```python
from build123d import *
from OCP.BRepFilletAPI import BRepFilletAPI_MakeChamfer

# Parameters (mm, degrees)
SKETCH2_R                = 12
BOSS_EXTRUDE1_DEPTH      = 81.85
SKETCH3_W                = 28.5
SKETCH3_H                = 57
SKETCH3_R                = 1.5
BOSS_EXTRUDE2_DEPTH      = 3
CHAMFER1_SIZE            = 1.5
SKETCH4_R                = 9.4
BOSS_EXTRUDE3_DEPTH      = 25.1
CUT_EXTRUDE1_DEPTH       = 88.8335642
CUT_EXTRUDE1_DEPTH_BACK  = 88.8335642
CHAMFER2_SIZE            = 2
CHAMFER2_SIZE2           = 2.066892656
CHAMFER3_SIZE            = 2
SKETCH6_R                = 4.5
CUT_EXTRUDE2_DEPTH       = 88.8335642
CUT_EXTRUDE2_DEPTH_BACK  = 88.8335642
SKETCH7_W                = 35.652875986
SKETCH7_H                = 43.298184849
SKETCH7_W_2              = 11
SKETCH7_H_2              = 30
CUT_EXTRUDE3_DEPTH       = 44
SKETCH8_R                = 4.5
BOSS_EXTRUDE4_DEPTH      = 2.5
BOSS_EXTRUDE4_DEPTH_BACK = 2.5
SKETCH9_R                = 3.5
CUT_EXTRUDE4_DEPTH       = 89.891703775


with BuildPart() as part:
    # Sketch2 → Boss-Extrude1 (new body)
    with BuildSketch(Plane.XY):
        Circle(SKETCH2_R)
    extrude(amount=-BOSS_EXTRUDE1_DEPTH)

    # Sketch3 → Boss-Extrude2 (add)
    with BuildSketch(Plane.XY):
        Rectangle(SKETCH3_W, SKETCH3_H)
        with Locations((0, 20.5)):
            Circle(SKETCH3_R, mode=Mode.SUBTRACT)
        with Locations((0, -20.5)):
            Circle(SKETCH3_R, mode=Mode.SUBTRACT)
    extrude(amount=BOSS_EXTRUDE2_DEPTH)

    # Chamfer1
    chamfer1_edges = [part.edges().sort_by_distance(p)[0] for p in [
        (-1.5, 20.5, 3),
        (-1.5, -20.5, 3),
    ]]
    chamfer(chamfer1_edges, length=CHAMFER1_SIZE)

    # Sketch4 → Boss-Extrude3 (add)
    with BuildSketch(Plane.XY.offset(3)):
        Circle(SKETCH4_R)
    extrude(amount=BOSS_EXTRUDE3_DEPTH)

    # Sketch5 → Cut-Extrude1 (cut, two sides)
    with BuildSketch(Plane(origin=(0, 0, 0), x_dir=(1, 0, 0), z_dir=(0, 1, 0))) as cut_extrude1_sk:
        Polygon((-7.85, -3), (-7.05, -28.1), (-9.4, -28.1), (-9.4, -3), align=None)
        Polygon((9.4, -3), (7.85, -3), (7.05, -28.1), (9.4, -28.1), align=None)
    extrude(amount=CUT_EXTRUDE1_DEPTH, mode=Mode.SUBTRACT)
    extrude(cut_extrude1_sk.sketch, amount=-CUT_EXTRUDE1_DEPTH_BACK, mode=Mode.SUBTRACT)

    # Chamfer2: one chamfer whose edges measure the first distance from different faces: ONE call of the kernel's chamfer builder (chamfer() names one face for all edges)
    chamfer2_edges_1 = [part.edges().sort_by_distance(p)[0] for p in [
        (0, -9.4, 28.1),
        (0, 9.4, 28.1),
    ]]
    chamfer2_edges_2 = [part.edges().sort_by_distance(p)[0] for p in [
        (7.05, 0, 28.1),
        (-7.05, 0, 28.1),
    ]]
    chamfer2_side_2 = [part.faces().sort_by_distance(p)[0] for p in [
        (0, 0, 28.1),
    ]]
    chamfer2 = BRepFilletAPI_MakeChamfer(part.part.solid().wrapped)
    for e in chamfer2_edges_1:
        chamfer2.Add(CHAMFER2_SIZE, e.wrapped)
    for e in chamfer2_edges_2:
        chamfer2.Add(CHAMFER2_SIZE, CHAMFER2_SIZE2, e.wrapped, chamfer2_side_2[0].wrapped)  # the first distance lies on this face
    add(Compound.cast(chamfer2.Shape()), mode=Mode.REPLACE)

    # Chamfer3
    chamfer3_edges = [part.edges().sort_by_distance(p)[0] for p in [
        (-12, 0, -81.85),
    ]]
    chamfer(chamfer3_edges, length=CHAMFER3_SIZE)

    # Sketch6 → Cut-Extrude2 (cut, two sides)
    with BuildSketch(Plane(origin=(0, 0, 0), x_dir=(0, 0, -1), z_dir=(1, 0, 0))) as cut_extrude2_sk:
        with Locations((57, -7)):
            Circle(SKETCH6_R)
    extrude(amount=CUT_EXTRUDE2_DEPTH, mode=Mode.SUBTRACT)
    extrude(cut_extrude2_sk.sketch, amount=-CUT_EXTRUDE2_DEPTH_BACK, mode=Mode.SUBTRACT)

    # Sketch7 → Cut-Extrude3 (cut)
    with BuildSketch(Plane(origin=(0, 0, -81.85), x_dir=(-1, 0, 0), z_dir=(0, 0, -1))):
        with Locations((0.794809337, 0.340632573)):
            Rectangle(SKETCH7_W, SKETCH7_H)
        Rectangle(SKETCH7_W_2, SKETCH7_H_2, mode=Mode.SUBTRACT)
    extrude(amount=-CUT_EXTRUDE3_DEPTH, mode=Mode.SUBTRACT)

    # Sketch8 → Boss-Extrude4 (add, two sides)
    with BuildSketch(Plane(origin=(0, 0, 0), x_dir=(0, 0, -1), z_dir=(1, 0, 0))) as boss_extrude4_sk:
        with Locations((57, -7)):
            Circle(SKETCH8_R)
        Polygon((55.9, -5.9), (55.9, -3.6), (58.1, -3.6), (58.1, -5.9), (60.4, -5.9), (60.4, -8.1), (58.1, -8.1), (58.1, -10.4), (55.9, -10.4), (55.9, -8.1), (53.6, -8.1), (53.6, -5.9), align=None, mode=Mode.SUBTRACT)
    extrude(amount=BOSS_EXTRUDE4_DEPTH)
    extrude(boss_extrude4_sk.sketch, amount=-BOSS_EXTRUDE4_DEPTH_BACK)

    # Sketch9 → Cut-Extrude4 (cut, through all)
    with BuildSketch(Plane(origin=(5.5, 0, 0), x_dir=(0, 0, -1), z_dir=(1, 0, 0))):
        with Locations(Location((44.65, -4, 0), (0, 0, 90))):
            Circle(SKETCH9_R)
        with Locations(Location((69.35, -4, 0), (0, 0, 90))):
            Circle(SKETCH9_R)
    extrude(amount=-CUT_EXTRUDE4_DEPTH, mode=Mode.SUBTRACT)


solid = part.part
```
Check sheet for the modelled part. Datum: model origin and axes. Units: mm. A direction names the side the tool comes from. Round coordinates to 2 decimals unless told otherwise and drop trailing zeros. Loops run counter-clockwise (first coordinate to the right, second up) from the corner with the lowest first, then second, coordinate; pieces in that order, holes last. Notation, with made-up numbers: (79.25, 13) - (100.25, 13) arc R38 cw to (100.25, 51) - close; hole circle Ø8 at (1.25, 42). An arc over 180 degrees is marked (long way). Answer as a JSON object with one key per item and string values. Group by question number.
Q1. Mould release check, pull along Y, two halves, no side actions. Record for faces 1 (the face through (-3.98, -2.54, -56.41)), 2 (the face through (-14.25, 0, 1)), 3 (the face through (0.1, 9.4, 14.4)): released by +Y, released by -Y, zero draft, split by the parting line, or undercut.
Q2. Gauge pin test, flat ends, axial feed: P1, Ø4, axis at x = -6, y = -4.5, coming from the -Z side; P2, Ø17, axis at y = -1.5, z = -59.5, coming from the -X side; P3, Ø3, axis at x = -6, z = -18, coming from the +Y side; P4, Ø1.8, axis at x = 1, y = -10, coming from the +Z side. Record the tip position at first contact, or that the pin passes through.
Q3. Set-up check for faces 4 (the face through (0, -7, -53.6)), 5 (the face through (-11.99, 0.53, -21.62)), 6 (the face through (-0.1, -9.4, 14.4)): record each of +Z, -Z, +X, -X, +Y, -Y from which the full face is reachable in a straight line by a thin tool's end or side.
Q4. Sectioned sample at A-A, the plane y = 20.5. Enter the section's corners in (x, z).
Q5. Sectioned sample at D-D, the plane z = -33.5. Enter the section's corners in (x, y), plus the area to 3 significant figures.
Q6. Sectioned sample at C-C, the plane x = 0. Count the separate pieces of the cut face and the enclosed holes in it, plus the area to 3 significant figures.
Q7. Sectioned sample at B-B, the plane z = -69.35. Enter the section's corners in (x, y), plus the area to 3 significant figures.
Q8. Scan lines: line 1 along Y through (x, z) = (0, 0.65); line 2 along Z through (x, y) = (-4.15, -7); line 3 along Z through (x, y) = (3, -4). Record each from-to range of solid material in increasing order. Write a range as [from, to].
Solution:
{
 "1": {"face 1": "undercut", "face 2": "zero draft", "face 3": "released by +Y"},
 "2": {"P1": "stops at z = -81.85", "P2": "stops at x = -5.5", "P3": "stops at y = 11.12", "P4": "stops at z = 26.35"},
 "3": {"face 4": "+X, -X", "face 5": "-Z", "face 6": "+Z, -Y"},
 "4": {"outline": "(-14.25, 0) - (-1.5, 0) - (-1.5, 1.5) - (-3, 3) - (-14.25, 3) - close; (1.5, 0) - (14.25, 0) - (14.25, 3) - (3, 3) - (1.5, 1.5) - close"},
 "5": {"outline": "circle Ø24 at (0, 0)", "area": "452 mm²"},
 "6": {"separate pieces": "3", "enclosed holes": "3", "area": "2,470 mm²"},
 "7": {"outline": "(-5.5, -10.67) arc R12 ccw to (5.5, -10.67) - (5.5, -7.5) - (-5.5, -7.5) - close; (-5.5, -0.5) - (5.5, -0.5) - (5.5, 10.67) arc R12 ccw to (-5.5, 10.67) - close", "area": "177 mm²"},
 "8": {"line 1": "y = [-28.5, -22], [-19, 19], [22, 28.5]", "line 2": "z = [-81.85, -71.15], [-67.55, -61.5], [-52.5, -46.45], [-42.85, 27.36]", "line 3": "z = [-81.85, -72.85], [-65.85, -60.35], [-53.65, -48.15], [-41.15, 28.1]"}
}
